Could you check a few things on this model? Use its own coordinates, in mm. A direction names the side the tool comes from. Round coordinates to 2 decimals unless told otherwise and drop trailing zeros. Write each loop counter-clockwise with the first axis right and the second up, starting at its lowest first coordinate (ties: lowest second). Pieces come first, ordered by that corner, then holes. Notation, with made-up numbers: (14, -22) - (37, -22) arc R9 ccw to (37, -17) - close; hole circle Ø2 at (82.25, -17). An arc over 180 degrees is marked (long way). Put each result on its own line as item: value.
from build123d import *

# Parameters (mm, degrees)
BOSS_EXTRUDE1_DEPTH = 10
SKETCH3_R           = 2.25
CUT_EXTRUDE1_DEPTH  = 35


with BuildPart() as part:
    # Sketch2 → Boss-Extrude1 (new body)
    with BuildSketch(Plane(origin=(0, 0, 0), x_dir=(1, 0, 0), z_dir=(0, 1, 0))):
        Polygon((-5, 0), (0, 0), (0, 25), (-29, 25), (-29, 55), (-26.5, 55), (-26.5, 57.5), (-29, 74.5), (-29, 75.5), (-26.5, 92.5), (-26.5, 95), (-34, 95), (-34, 20), (-5, 20), align=None)
    extrude(amount=BOSS_EXTRUDE1_DEPTH)

    # Sketch3 → Cut-Extrude1 (cut, through all)
    with BuildSketch(Plane(origin=(0, 0, 0), x_dir=(0, 0, -1), z_dir=(1, 0, 0))):
        with Locations((3.5, 5)):
            Circle(SKETCH3_R)
        with Locations((12.5, 5)):
            Circle(SKETCH3_R)
    extrude(amount=-CUT_EXTRUDE1_DEPTH, mode=Mode.SUBTRACT)


solid = part.part
(1) Imagine slicing it at C-C, the plane z = -16.5. List the corners of the cut face in (x, y) for me.
Values found:
outline: (-5, 0) - (0, 0) - (0, 10) - (-5, 10) - close
(2) I'm going to push flat-ended pins straight in: pin 1 (2 mm diameter, centred on y = 6.5, z = -94, fed in from +X); pin 2 (2 mm diameter, centred on y = 5.5, z = -32.5, fed in from +X); pin 3 (4 mm diameter, centred on y = 5, z = -12.5, fed in from +X); pin 4 (5 mm diameter, centred on x = -10.5, y = 1.5, fed in from +Z). Where does each tip first touch, or does it pass through?
Values found:
pin 1: stops at x = -26.5
pin 2: stops at x = -29
pin 3: passes through
pin 4: stops at z = -20
(3) Please list where these lines run through material, in increasing order: probe 1 along Y at (x, z) = (-1.85, -3.5); probe 2 along X at (y, z) = (6.75, -35); probe 3 along Z at (x, y) = (-2, 9.75). Write a range as from..to.
Values found:
probe 1: y = 0..2.75, 7.25..10
probe 2: x = -34..-29
probe 3: z = -25..0
(4) For faces 4 (the face through (-2.46, 7.23, -3.21)), 5 (the face through (-26.5, 5, -56)), 6 (the face through (-29, 5, -40)), which set-ups out of +Z, -Z, +X, -X, +Y, -Y let a thin tool reach every point of the face, with its end or its side?
Values found:
face 4: +X, -X
face 5: -Z, +X, +Y, -Y
face 6: +X, +Y, -Y
(5) Imagine slicing it at B-B, the plane y = 5. List the corners of the cut face in (x, z) for me.
Values found:
outline: (-34, -95) - (-26.5, -95) - (-26.5, -92.5) - (-29, -75.5) - (-29, -74.5) - (-26.5, -57.5) - (-26.5, -55) - (-29, -55) - (-29, -25) - (0, -25) - (0, -14.75) - (-5, -14.75) - (-5, -20) - (-34, -20) - close; (-5, -10.25) - (0, -10.25) - (0, -5.75) - (-5, -5.75) - close; (-5, -1.25) - (0, -1.25) - (0, 0) - (-5, 0) - close
(6) If we mould it in two halves opening along Z, with no side actions, what happens to faces 1 (the face through (-27.768, 4.93, -83.881)), 2 (the face through (-5, 5, -10)), 3 (the face through (-20, 5, -20))? For each: pulls with the +Z half, pulls with the -Z half, needs draft (parallel to the pull), parting line crosses it, or undercut.
Values found:
face 1: undercut
face 2: needs draft
face 3: pulls with the +Z half
(7) Imagine slicing it at D-D, the plane x = -10. List the corners of the cut face in (y, z) for me.
Values found:
outline: (0, -25) - (10, -25) - (10, -20) - (0, -20) - close
(8) Imagine slicing it at A-A, the plane z = -3.5. List the corners of the cut face in (x, y) for me.
Values found:
outline: (-5, 0) - (0, 0) - (0, 2.75) - (-5, 2.75) - close; (-5, 7.25) - (0, 7.25) - (0, 10) - (-5, 10) - close
